from build123d import *
from build123d.topology import SkipClean

# Parameters (mm, degrees)
SKETCH1_R                 = 1.1557
BOSS_EXTRUDE1_DEPTH       = 0.7366
BOSS_EXTRUDE2_START       = 3.175
SKETCH2_R                 = 1.651
SKETCH2_R_2               = 1.1557
BOSS_EXTRUDE2_DEPTH       = 3.175
BOSS_EXTRUDE3_START       = -3.9116
SKETCH1_2_R               = 1.1557
BOSS_EXTRUDE3_DEPTH       = 0.7366
BOSS_EXTRUDE4_START       = -5.3848
SKETCH1_3_R               = 1.1557
BOSS_EXTRUDE4_DEPTH       = 0.7366
BOSS_EXTRUDE5_START       = 9.2964
SKETCH2_2_R               = 1.651
SKETCH2_2_R_2             = 1.1557
BOSS_EXTRUDE5_DEPTH       = 3.175
BOSS_EXTRUDE6_START       = -10.033
SKETCH1_4_R               = 1.1557
BOSS_EXTRUDE6_DEPTH       = 0.7366
BOSS_EXTRUDE7_DEPTH       = 0.7366
BOSS_EXTRUDE8_START       = -6.1214
BOSS_EXTRUDE8_DEPTH       = 1.4732
BOSS_EXTRUDE9_START       = -11.5062
BOSS_EXTRUDE9_DEPTH       = 0.7366
BOSS_EXTRUDE10_DEPTH      = 0.7366
BOSS_EXTRUDE10_DEPTH_BACK = 12.9794
SKETCH4_R                 = 1.1557


with BuildPart() as part:
    # Sketch1 → Boss-Extrude1 (new body)
    with BuildSketch(Plane.XY):
        with BuildLine():
            ThreePointArc((-1.5875, 2.421640582), (-6.0706, 0), (-1.5875, -2.421640582))
            ThreePointArc((-1.5875, -2.421640582), (0, -1.947681165), (1.5875, -2.421640582))
            ThreePointArc((1.5875, -2.421640582), (6.0706, 0), (1.5875, 2.421640582))
            ThreePointArc((1.5875, 2.421640582), (0, 1.947681165), (-1.5875, 2.421640582))
        make_face()
        with Locations((-3.175, 0)):
            Circle(SKETCH1_R, mode=Mode.SUBTRACT)
        with Locations((3.175, 0)):
            Circle(SKETCH1_R, mode=Mode.SUBTRACT)
    extrude(amount=BOSS_EXTRUDE1_DEPTH)

    # Sketch2 → Boss-Extrude2 (add)
    # profile 1 of 2: a face of its own
    with SkipClean():  # the faces are left unmerged after this step: merging them gives an invalid solid
        with BuildSketch(Plane(origin=(0, 0, 0), x_dir=(-1, 0, 0), z_dir=(0, 0, -1)).offset(BOSS_EXTRUDE2_START)):
            with Locations(Location((3.175, 0, 0), (0, 0, 180))):
                Circle(SKETCH2_R)
            with Locations((3.175, 0)):
                Circle(SKETCH2_R_2, mode=Mode.SUBTRACT)
        # profile 2 of 2: a face of its own
        with BuildSketch(Plane(origin=(0, 0, 0), x_dir=(-1, 0, 0), z_dir=(0, 0, -1)).offset(BOSS_EXTRUDE2_START)):
            with Locations(Location((-3.175, 0, 0), (0, 0, 180))):
                Circle(SKETCH2_R)
            with Locations((-3.175, 0)):
                Circle(SKETCH2_R_2, mode=Mode.SUBTRACT)
        extrude(amount=-BOSS_EXTRUDE2_DEPTH)

    # Sketch1<2> → Boss-Extrude3 (add)
    with SkipClean():  # the faces are left unmerged after this step: merging them gives an invalid solid
        with BuildSketch(Plane.XY.offset(BOSS_EXTRUDE3_START)):
            with BuildLine():
                ThreePointArc((-1.5875, 2.421640582), (-6.0706, 0), (-1.5875, -2.421640582))
                ThreePointArc((-1.5875, -2.421640582), (0, -1.947681165), (1.5875, -2.421640582))
                ThreePointArc((1.5875, -2.421640582), (6.0706, 0), (1.5875, 2.421640582))
                ThreePointArc((1.5875, 2.421640582), (0, 1.947681165), (-1.5875, 2.421640582))
            make_face()
            with Locations(Location((-3.175, 0, 0), (0, 0, 180))):
                Circle(SKETCH1_2_R, mode=Mode.SUBTRACT)
            with Locations(Location((3.175, 0, 0), (0, 0, 180))):
                Circle(SKETCH1_2_R, mode=Mode.SUBTRACT)
        extrude(amount=BOSS_EXTRUDE3_DEPTH)

    # Sketch3 → Boss-Extrude7 (add)
    with SkipClean():  # the faces are left unmerged after this step: merging them gives an invalid solid
        with BuildSketch(Plane.XY.offset(0.7366)):
            with BuildLine():
                ThreePointArc((4.645703355, 2.020063927), (0.676275, 0), (4.645703355, -2.020063927))
                ThreePointArc((4.645703355, -2.020063927), (6.35, -1.465376634), (8.054296645, -2.020063927))
                ThreePointArc((8.054296645, -2.020063927), (12.023725, 0), (8.054296645, 2.020063927))
                ThreePointArc((8.054296645, 2.020063927), (6.35, 1.465376634), (4.645703355, 2.020063927))
            make_face()
        extrude(amount=BOSS_EXTRUDE7_DEPTH)



with BuildPart() as body_2:
    # Sketch1<3> → Boss-Extrude4 (new body)
    with BuildSketch(Plane.XY.offset(BOSS_EXTRUDE4_START)):
        with BuildLine():
            ThreePointArc((-1.5875, 2.421640582), (-6.0706, 0), (-1.5875, -2.421640582))
            ThreePointArc((-1.5875, -2.421640582), (0, -1.947681165), (1.5875, -2.421640582))
            ThreePointArc((1.5875, -2.421640582), (6.0706, 0), (1.5875, 2.421640582))
            ThreePointArc((1.5875, 2.421640582), (0, 1.947681165), (-1.5875, 2.421640582))
        make_face()
        with Locations(Location((-3.175, 0, 0), (0, 0, 180))):
            Circle(SKETCH1_3_R, mode=Mode.SUBTRACT)
        with Locations(Location((3.175, 0, 0), (0, 0, 180))):
            Circle(SKETCH1_3_R, mode=Mode.SUBTRACT)
    extrude(amount=-BOSS_EXTRUDE4_DEPTH)

    # Sketch2<2> → Boss-Extrude5 (add)
    # profile 1 of 2: a face of its own
    with BuildSketch(Plane(origin=(0, 0, 0), x_dir=(-1, 0, 0), z_dir=(0, 0, -1)).offset(BOSS_EXTRUDE5_START)):
        with Locations((3.175, 0)):
            Circle(SKETCH2_2_R)
        with Locations((3.175, 0)):
            Circle(SKETCH2_2_R_2, mode=Mode.SUBTRACT)
    # profile 2 of 2: a face of its own
    with BuildSketch(Plane(origin=(0, 0, 0), x_dir=(-1, 0, 0), z_dir=(0, 0, -1)).offset(BOSS_EXTRUDE5_START)):
        with Locations((-3.175, 0)):
            Circle(SKETCH2_2_R)
        with Locations((-3.175, 0)):
            Circle(SKETCH2_2_R_2, mode=Mode.SUBTRACT)
    extrude(amount=-BOSS_EXTRUDE5_DEPTH)

    # Sketch1<4> → Boss-Extrude6 (add)
    with BuildSketch(Plane.XY.offset(BOSS_EXTRUDE6_START)):
        with BuildLine():
            ThreePointArc((-1.5875, 2.421640582), (-6.0706, 0), (-1.5875, -2.421640582))
            ThreePointArc((-1.5875, -2.421640582), (0, -1.947681165), (1.5875, -2.421640582))
            ThreePointArc((1.5875, -2.421640582), (6.0706, 0), (1.5875, 2.421640582))
            ThreePointArc((1.5875, 2.421640582), (0, 1.947681165), (-1.5875, 2.421640582))
        make_face()
        with Locations(Location((-3.175, 0, 0), (0, 0, 180))):
            Circle(SKETCH1_4_R, mode=Mode.SUBTRACT)
        with Locations(Location((3.175, 0, 0), (0, 0, 180))):
            Circle(SKETCH1_4_R, mode=Mode.SUBTRACT)
    extrude(amount=BOSS_EXTRUDE6_DEPTH)


with BuildPart() as part_1:
    with SkipClean():  # the faces are left unmerged after this step: merging them gives an invalid solid
        add(part.part)

        add(body_2.part)  # Boss-Extrude8 merges body 2
        # Sketch3<2> → Boss-Extrude8 (add)
        with BuildSketch(Plane.XY.offset(0.7366).offset(BOSS_EXTRUDE8_START)):
            with BuildLine():
                ThreePointArc((4.645703355, 2.020063927), (0.676275, 0), (4.645703355, -2.020063927))
                ThreePointArc((4.645703355, -2.020063927), (6.35, -1.465376634), (8.054296645, -2.020063927))
                ThreePointArc((8.054296645, -2.020063927), (12.023725, 0), (8.054296645, 2.020063927))
                ThreePointArc((8.054296645, 2.020063927), (6.35, 1.465376634), (4.645703355, 2.020063927))
            make_face()
        extrude(amount=BOSS_EXTRUDE8_DEPTH)

    # Sketch3<3> → Boss-Extrude9 (add)
    with BuildSketch(Plane.XY.offset(0.7366).offset(BOSS_EXTRUDE9_START)):
        with BuildLine():
            ThreePointArc((4.645703355, 2.020063927), (0.676275, 0), (4.645703355, -2.020063927))
            ThreePointArc((4.645703355, -2.020063927), (6.35, -1.465376634), (8.054296645, -2.020063927))
            ThreePointArc((8.054296645, -2.020063927), (12.023725, 0), (8.054296645, 2.020063927))
            ThreePointArc((8.054296645, 2.020063927), (6.35, 1.465376634), (4.645703355, 2.020063927))
        make_face()
    extrude(amount=BOSS_EXTRUDE9_DEPTH)

    # Sketch4 → Boss-Extrude10 (add, two sides: drawn at the far end of the back side and taken through both)
    with BuildSketch(Plane.XY.offset(1.4732).offset(-BOSS_EXTRUDE10_DEPTH_BACK)):
        with Locations(Location((3.175, 0, 0), (0, 0, 180))):
            Circle(SKETCH4_R)
        with Locations(Location((9.525, 0, 0), (0, 0, 180))):
            Circle(SKETCH4_R)
    extrude(amount=BOSS_EXTRUDE10_DEPTH + BOSS_EXTRUDE10_DEPTH_BACK)


solid = part_1.part
Geometry check sheet. Reference: the model listing, model coordinates, mm. A direction names the side the tool comes from. Coordinates: 2 decimals unless noted, no trailing zeros. Order: outer loops, then holes, each group sorted by start corner. A loop starts at its lowest first (then second) coordinate and runs counter-clockwise, first axis right, second up. Notation, with made-up numbers: (-30.5, 29) -> (-9.5, 29) arc R15 ccw to (-9.5, 55) -> close; hole circle Ø1 at (31, -37). An arc over 180 degrees is marked (long way). Use a Markdown table: item, result. Add a question column.
1. Mould release check, pull along Z, two halves, no side actions. Record for faces 1 (the face through (-1.6, 0, 0.737)), 2 (the face through (-1.6, 0, -10.033)), 3 (the face through (-1.6, -0.5, -1.6)): pulls with the +Z half, pulls with the -Z half, needs draft (parallel to the pull), parting line crosses it, or undercut.
2. Cross-section at B-B (y = 0). Give the number of separate pieces and of enclosed holes in the cut face, and give its area (3 significant figures).
3. Cross-section at C-C (x = 1.25). Enter the section's corners in (y, z) (3 decimals).
4. Go/stop test with flat-tipped pins: pin 1 Ø1.7 at (x, y) = (-2, 0) entering from -Z; pin 2 Ø3 at (x, y) = (-0.5, 1) entering from +Z; pin 3 Ø1 at (x, z) = (7.5, -10) entering from -Y; pin 4 Ø3 at (x, z) = (-2.5, -1) entering from -Y. Record where each tip stops, or that it passes through.
5. Cross-section at D-D (z = -10.5). Enter the section's corners in (x, y) (3 decimals), and give its area (3 significant figures).
6. Material ranges on L1, parallel to Z at x = 3.25, y = 2.05 (3 decimals); L2, parallel to Z at x = 6.75, y = 0.9; L3, parallel to Z at x = 5, y = 2.1 (3 decimals), recorded low to high.
7. Cross-section at A-A (z = -2). Enter the section's corners in (x, y) (3 decimals).
8. Set-up check for faces 4 (the face through (10.68, -0.05, 1.84)), 5 (the face through (6, 0, -10.77)), 6 (the face through (10.68, -0.05, -1.62)): record each of +Z, -Z, +X, -X, +Y, -Y from which the full face is reachable in a straight line by a thin tool's end or side.
Filled sheet:
| question | item | result |
|---|---|---|
| 1 | face 1 | pulls with the +Z half |
| 1 | face 2 | pulls with the -Z half |
| 1 | face 3 | undercut |
| 2 | separate pieces | 3 |
| 2 | enclosed holes | 4 |
| 2 | area | 118 mm2 |
| 3 | outline | (-2.231, -10.033) -> (-1.593, -10.033) -> (-1.593, -10.77) -> (1.593, -10.77) -> (1.593, -10.033) -> (2.231, -10.033) -> (2.231, -9.296) -> (-2.231, -9.296) -> close; (-2.231, -6.121) -> (2.231, -6.121) -> (2.231, -5.385) -> (1.593, -5.385) -> (1.593, -3.912) -> (2.231, -3.912) -> (2.231, -3.175) -> (-2.231, -3.175) -> (-2.231, -3.912) -> (-1.593, -3.912) -> (-1.593, -5.385) -> (-2.231, -5.385) -> close; (-2.231, 0) -> (2.231, 0) -> (2.231, 0.737) -> (1.593, 0.737) -> (1.593, 1.473) -> (-1.593, 1.473) -> (-1.593, 0.737) -> (-2.231, 0.737) -> close |
| 4 | pin 1 | z = -10.03 |
| 4 | pin 2 | z = 1.47 |
| 4 | pin 3 | y = -1.98 |
| 4 | pin 4 | y = -2.9 |
| 5 | outline | (4.646, -2.02) arc R2.896 cw to (8.054, -2.02) arc R2.499 ccw (long way) to (8.054, 2.02) arc R2.896 cw to (4.646, 2.02) arc R2.499 ccw (long way) to start |
| 5 | area | 44.6 mm2 |
| 6 | L1 | -10.77 to -9.296, -6.121 to -3.175, 0 to 1.473 |
| 6 | L2 | -10.77 to -10.03, -5.38 to -3.91, 0.74 to 1.47 |
| 6 | L3 | -10.033 to -9.296, -6.121 to -5.385, -3.912 to -3.175, 0 to 0.737 |
| 7 | outline | circle Ø3.302 at (-3.175, 0); circle Ø3.302 at (3.175, 0); circle Ø2.311 at (9.525, 0); hole circle Ø2.311 at (-3.175, 0) |
| 8 | face 4 | +Z |
| 8 | face 5 | -Z |
| 8 | face 6 | none |
